Build history of the part. All positions in model axes, mm. Face numbers are marked on the shaded views. A direction names the side the tool comes from. Round coordinates to 2 decimals unless told otherwise and drop trailing zeros. Write each loop counter-clockwise with the first axis right and the second up, starting at its lowest first coordinate (ties: lowest second). Pieces come first, ordered by that corner, then holes.
Item 1: Wall check: probe 1 along X at (y, z) = (-20, 19.5); probe 2 along X at (y, z) = (-35, 13.5). Give the ranges that are in metal, low to high.
Item 2: Band-saw the part on B-B, the plane y = -5. Write the cut outline in (x, z).
Item 3: Band-saw the part on C-C, the plane x = -21.5. Write the cut outline in (y, z).
Item 4: 3-axis set-ups, long thin cutter, end or side, ignore diameter. For the marked faces 4, 5 and 6: which of +Z, -Z, +X, -X, +Y, -Y reach the whole face in a straight line?
Item 5: Band-saw the part on A-A, the plane z = 13.5. Write the cut outline in (x, y).
Item 6: Drop flat-ended pins along their axis: pin 1 Ø3 at (y, z) = (-37, 26.5) entering from -X; pin 2 Ø2.5 at (y, z) = (-4.5, 29) entering from -X; pin 3 Ø2.5 at (x, z) = (-32, 6) entering from -Y. Give the stop position or say it passes through.
Item 7: Mould opens along X. For the marked faces 1, 2 and 3 say: +X half, -X half, draft (parallel to the pull), parting line (faces both ways), or undercut.
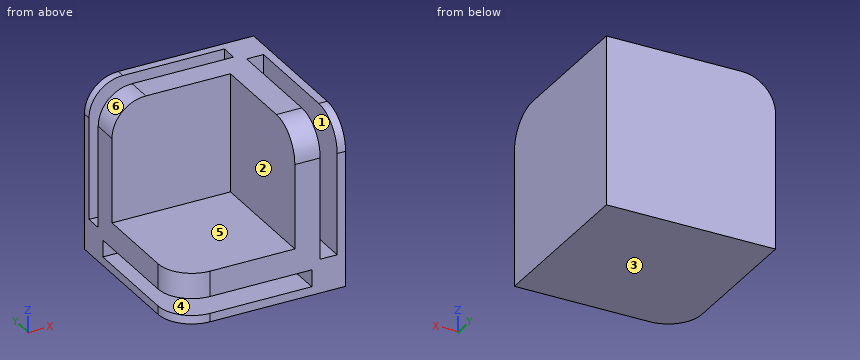
```python
from build123d import *

# Parameters (mm, degrees)
F1_DEPTH = 15
F3_DEPTH = 15
F5_DEPTH = 15
F6_W     = 20
F6_H     = 5
F6_W_2   = 5
F6_H_2   = 30
F6_H_3   = 20
F7_DEPTH = 40
F8_W     = 30
F8_H     = 5
F8_W_2   = 20
F9_DEPTH = 40


# Not quite as in the source:
# - a feature names something its author has since deleted; it is built from what else it names


with BuildPart() as f1:
    # F0 (on Top) → F1 (new body)
    with BuildSketch(Plane.XY):
        with BuildLine():
            Line((0, -50), (0, 0))
            Line((0, 0), (-50, 0))
            Line((-50, 0), (-50, -40))
            ThreePointArc((-50, -40), (-47.0710678119, -47.0710678119), (-40, -50))
            Line((-40, -50), (0, -50))
        make_face()
    extrude(amount=F1_DEPTH)

    # F2 (on Right) → F3 (join)
    with BuildSketch(Plane.YZ):
        with BuildLine():
            Line((-50, 10), (0, 10))
            Line((0, 10), (0, 50))
            Line((0, 50), (-40, 50))
            ThreePointArc((-40, 50), (-47.0710678119, 47.0710678119), (-50, 40))
            Line((-50, 40), (-50, 10))
        make_face()
    extrude(amount=-F3_DEPTH)

    # F4 (on Front) → F5 (join)
    with BuildSketch(Plane.XZ):
        with BuildLine():
            Line((-50, 10), (-10, 10))
            Line((-10, 10), (-10, 50))
            Line((-10, 50), (-40, 50))
            ThreePointArc((-40, 50), (-47.0710678119, 47.0710678119), (-50, 40))
            Line((-50, 40), (-50, 10))
        make_face()
    extrude(amount=F5_DEPTH)

    # F6 (on face) → F7 (cut)
    with BuildSketch(Plane.XZ.offset(50)):
        Polygon((-15, 2.5), (-10, 2.5), (-10, 7.5), (-40, 7.5), (-40, 2.5), align=None)
        with Locations((-50, 5)):
            Rectangle(F6_W, F6_H)
        with Locations((-5, 25)):
            Rectangle(F6_W_2, F6_H_2)
        with Locations((-5, 50)):
            Rectangle(F6_W_2, F6_H_3)
    extrude(amount=-F7_DEPTH, mode=Mode.SUBTRACT)

    # F8 (on face) → F9 (cut)
    with BuildSketch(Plane.XY.offset(50)):
        with Locations((-25, -5)):
            Rectangle(F8_W, F8_H)
        with Locations((-50, -5)):
            Rectangle(F8_W_2, F8_H)
    extrude(amount=-F9_DEPTH, mode=Mode.SUBTRACT)


solid = f1.part
```
Results:
1. probe 1: x = -15 to -7.5, -2.5 to 0
1. probe 2: x = -50 to -7.5, -2.5 to 0
2. outline: (-50, 0) - (0, 0) - (0, 50) - (-10, 50) - (-10, 10) - (-50, 10) - close
3. outline: (-50, 0) - (0, 0) - (0, 50) - (-2.5, 50) - (-2.5, 10) - (-7.5, 10) - (-7.5, 50) - (-15, 50) - (-15, 15) - (-50, 15) - (-50, 7.5) - (-10, 7.5) - (-10, 2.5) - (-50, 2.5) - close
4. face 4: -X, -Y
4. face 5: +Z, -X, -Y
4. face 6: +Z, -X, +Y, -Y
5. outline: (-50, -40) arc R10 ccw to (-40, -50) - (-7.5, -50) - (-7.5, -10) - (-2.5, -10) - (-2.5, -50) - (0, -50) - (0, 0) - (-50, 0) - (-50, -2.5) - (-10, -2.5) - (-10, -7.5) - (-50, -7.5) - close
6. pin 1: stops at x = -15
6. pin 2: stops at x = -10
6. pin 3: stops at y = -10
7. face 1: undercut
7. face 2: -X half
7. face 3: draft
